from build123d import *

# Parameters (mm, degrees)
SKETCH1_W           = 38.1
SKETCH1_H           = 25.4
SKETCH1_R           = 3.175
BOSS_EXTRUDE1_DEPTH = 25.4
SKETCH2_R           = 9.525
SKETCH2_R_2         = 5.55625
CUT_EXTRUDE1_DEPTH  = 23.495
SKETCH2_4_R         = 5.55625
CUT_EXTRUDE2_DEPTH  = 48.519048865
FILLET1_DEPTH       = 25.4
FILLET2_R           = 2.116666667


with BuildPart() as part:
    # Sketch1 → Boss-Extrude1 (new body)
    with BuildSketch(Plane.XY):
        with Locations((-6.35, 0)):
            Rectangle(SKETCH1_W, SKETCH1_H)
        Circle(SKETCH1_R, mode=Mode.SUBTRACT)
    extrude(amount=BOSS_EXTRUDE1_DEPTH)

    # Sketch2 → Cut-Extrude1 (cut)
    # profile 1 of 2: a face of its own
    with BuildSketch(Plane(origin=(12.7, 0, 0), x_dir=(0, 0, -1), z_dir=(1, 0, 0))):
        with Locations(Location((-12.7, 0, 0), (0, 0, 90))):
            Circle(SKETCH2_R)
        with Locations((-12.7, 0)):
            Circle(SKETCH2_R_2, mode=Mode.SUBTRACT)
    # profile 2 of 2: a face of its own
    with BuildSketch(Plane(origin=(12.7, 0, 0), x_dir=(0, 0, -1), z_dir=(1, 0, 0))):
        with Locations((-12.7, 0)):
            Circle(SKETCH2_R_2)
    extrude(amount=-CUT_EXTRUDE1_DEPTH, mode=Mode.SUBTRACT)

    # Sketch2<4> → Cut-Extrude2 (cut, through all)
    with BuildSketch(Plane(origin=(12.7, 0, 0), x_dir=(0, 0, -1), z_dir=(1, 0, 0))):
        with Locations(Location((-12.7, 0, 0), (0, 0, 90))):
            Circle(SKETCH2_4_R)
    extrude(amount=-CUT_EXTRUDE2_DEPTH, mode=Mode.SUBTRACT)

    # Fillet1: read off the stored shape, not the designer's step
    # Fillet1 outline → Fillet1 (cut)
    with BuildSketch(Plane.XY):
        with BuildLine():
            Line((12.7, 12.7), (0, 12.7))
            ThreePointArc((0, 12.7), (8.980256121, 8.980256121), (12.7, 0))
            Line((12.7, 0), (12.7, 12.7))
        make_face()
        with BuildLine():
            Line((12.7, -12.7), (12.7, 0))
            ThreePointArc((12.7, 0), (8.980256121, -8.980256121), (0, -12.7))
            Line((0, -12.7), (12.7, -12.7))
        make_face()
    extrude(amount=FILLET1_DEPTH, mode=Mode.SUBTRACT)

    # Fillet2
    fillet2_edges = [part.edges().sort_by_distance(p)[0] for p in [
        (-25.4, 0, 25.4),
        (-12.7, -12.7, 25.4),
        (-12.7, 12.7, 0),
        (8.980256121, 8.980256121, 0),
        (8.980256121, -8.980256121, 0),
        (-12.7, 12.7, 25.4),
        (8.980256121, 8.980256121, 25.4),
        (8.980256121, -8.980256121, 25.4),
        (-12.7, -12.7, 0),
        (-25.4, 0, 0),
        (-25.4, -12.7, 12.7),
        (-25.4, 12.7, 12.7),
    ]]
    fillet(fillet2_edges, radius=FILLET2_R)


solid = part.part
Work out the finished part from the listing and answer in its coordinate system (mm). A direction names the side the tool comes from. Round coordinates to 2 decimals unless told otherwise and drop trailing zeros. Write each loop counter-clockwise with the first axis right and the second up, starting at its lowest first coordinate (ties: lowest second). Pieces come first, ordered by that corner, then holes. Notation, with made-up numbers: M 3.5,28.5 L 9.5,28.5 A19 cw 9.5,60.5 Z; hole C -12.5,69 d7. An arc over 180 degrees is marked long. Use a Markdown table: item, result.
1) The part is cut by section A-A on x = -15.5. Give the vertices of the cut face in (y, z), plus the area to 3 significant figures.
Taken from the geometry:
| item | result |
|---|---|
| outline | M -12.7,2.12 A2.12 ccw -10.58,0 L 10.58,0 A2.12 ccw 12.7,2.12 L 12.7,23.28 A2.12 ccw 10.58,25.4 L -10.58,25.4 A2.12 ccw -12.7,23.28 Z; hole C 0,12.7 d11.11 |
| area | 544 mm2 |
2) The part is cut by section D-D on y = 2.25. State how many separate pieces and enclosed holes the cut face has, plus the area to 3 significant figures.
Taken from the geometry:
| item | result |
|---|---|
| separate pieces | 4 |
| enclosed holes | 0 |
| area | 348 mm2 |
3) Consider line 1 (Y direction, x = 0, z = 2.4) (3 decimals); line 2 (Z direction, x = -4.25, y = 0) (3 decimals); line 3 (Z direction, x = -15, y = 0). Determine where each line is inside the solid, lowest interval first. Write a range as [from, to].
Taken from the geometry:
| item | result |
|---|---|
| line 1 | y = [-12.7, -3.175], [3.175, 12.7] |
| line 2 | z = [0, 3.175], [22.225, 25.4] |
| line 3 | z = [0, 7.14], [18.26, 25.4] |
4) The part is cut by section C-C on z = 5.25. Give the vertices of the cut face in (x, y) (3 decimals), plus the area to 3 significant figures.
Taken from the geometry:
| item | result |
|---|---|
| outline | M -25.4,-10.583 A2.117 ccw -23.283,-12.7 L 0,-12.7 A12.7 ccw 11.228,-5.935 L -10.795,-5.935 L -10.795,5.935 L 11.228,5.935 A12.7 ccw 0,12.7 L -23.283,12.7 A2.117 ccw -25.4,10.583 Z |
| area | 623 mm2 |
5) The part is cut by section B-B on z = 14. Give the vertices of the cut face in (x, y) (3 decimals), plus the area to 3 significant figures.
Taken from the geometry:
| item | result |
|---|---|
| outline | M -25.4,-10.583 A2.117 ccw -23.283,-12.7 L 0,-12.7 A12.7 ccw 8.5,-9.436 L -10.795,-9.436 L -10.795,-5.402 L -25.4,-5.402 Z; M -25.4,5.402 L -10.795,5.402 L -10.795,9.436 L 8.5,9.436 A12.7 ccw 0,12.7 L -23.283,12.7 A2.117 ccw -25.4,10.583 Z |
| area | 320 mm2 |
6) Flat-ended cylindrical pins translate along their axes: pin 1 (12 mm diameter, centred on x = 8, z = 20, fed in from +Y); pin 2 (15 mm diameter, centred on y = -4.5, z = 16, fed in from +X); pin 3 (6 mm diameter, centred on x = 3.5, z = 4, fed in from +Y). Find the tip coordinate at first contact, or state that the pin passes through.
Taken from the geometry:
| item | result |
|---|---|
| pin 1 | stops at y = 12.54 |
| pin 2 | stops at x = 12.7 |
| pin 3 | stops at y = 12.69 |
7) Determine the mould class of faces 1 (the face through (-7, 0, 25.4)), 2 (the face through (-18, -0.72, 18.21)), 3 (the face through (-11.8, 12.1, 24.76)) for opening direction Y: pulls with the +Y half, pulls with the -Y half, needs draft (parallel to the pull), parting line crosses it, or undercut.
Taken from the geometry:
| item | result |
|---|---|
| face 1 | needs draft |
| face 2 | undercut |
| face 3 | pulls with the +Y half |
8) Which of the six approach directions +Z, -Z, +X, -X, +Y, -Y give full straight-line access (tool end or side, diameter ignored) to faces 4 (the face through (1.12, 8.8, 9.05)), 5 (the face through (3.03, 0.95, 1.84))?
Taken from the geometry:
| item | result |
|---|---|
| face 4 | +X |
| face 5 | +Z, -Z |
